Can you work these out from the drawing? Everything is in mm from the part's minimum corner. A direction names the side the tool comes from. Round coordinates to 2 decimals unless told otherwise and drop trailing zeros. Write each loop counter-clockwise with the first axis right and the second up, starting at its lowest first coordinate (ties: lowest second). Pieces come first, ordered by that corner, then holes. Notation, with made-up numbers: (-20.5, 81.25) - (-1.5, 81.25) arc R9 cw to (-1.5, 98.25) - close; hole circle Ø9 at (50.25, 70). An arc over 180 degrees is marked (long way). One line per item, written item: value. Start each with the question number.
Item 1: Imagine slicing it at B-B, the plane x = 53.5. Please give me the cut outline in (y, z), then the cut area to 4 significant figures.
Item 2: For P1, Ø1.5, axis at x = 64, y = 88.5, coming from the +Z side; P2, Ø5, axis at y = 11.5, z = 62, coming from the +X side (1 decimal); P3, Ø20.5, axis at x = 128.5, y = 65.5, coming from the +Z side, each with a flat end and sliding along its axis, tell me the tip position at first contact or that it passes through.
Item 3: Imagine slicing it at C-C, the plane z = 80. Please give me the cut outline in (x, y) (1 decimal).
Item 4: For the marked faces 1 and 2, which set-ups out of +Z, -Z, +X, -X, +Y, -Y let a thin tool reach every point of the face, with its end or its side?
Item 5: If I drill on line 1 (Z direction, x = 133.5, y = 59); line 2 (Z direction, x = 48.5, y = 83); line 3 (X direction, y = 26, z = 79) (1 decimal), over which ranges is the centre line in solid material (lowest first)?
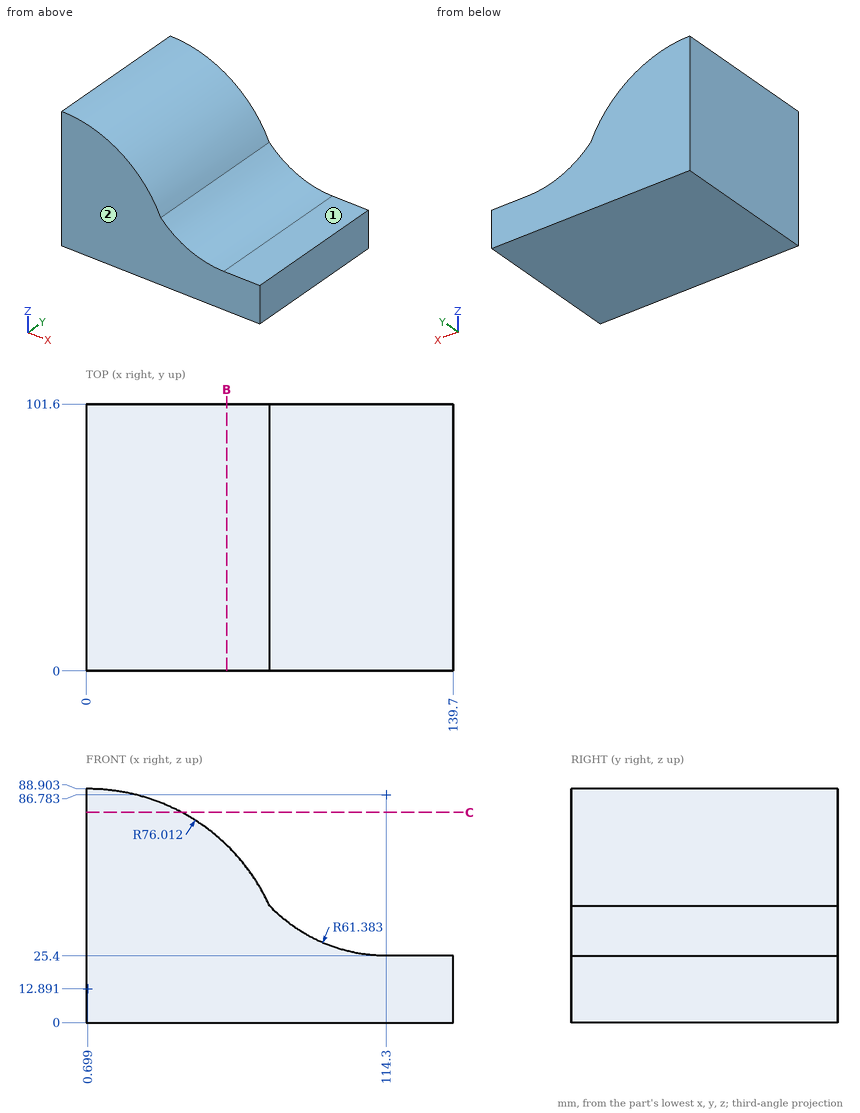
Values follow:
1. outline: (0, 0) - (101.6, 0) - (101.6, 67.57) - (0, 67.57) - close
1. area: 6,865 mm^2
2. P1: stops at z = 56.08
2. P2: stops at x = 60.7
2. P3: stops at z = 25.4
3. outline: (0, 0) - (36.4, 0) - (36.4, 101.6) - (0, 101.6) - close
4. face 1: +Z, +X, +Y, -Y
4. face 2: +Z, -Z, +X, -X, -Y
5. line 1: z = 0 to 25.4
5. line 2: z = 0 to 71.99
5. line 3: x = 0 to 38.2
